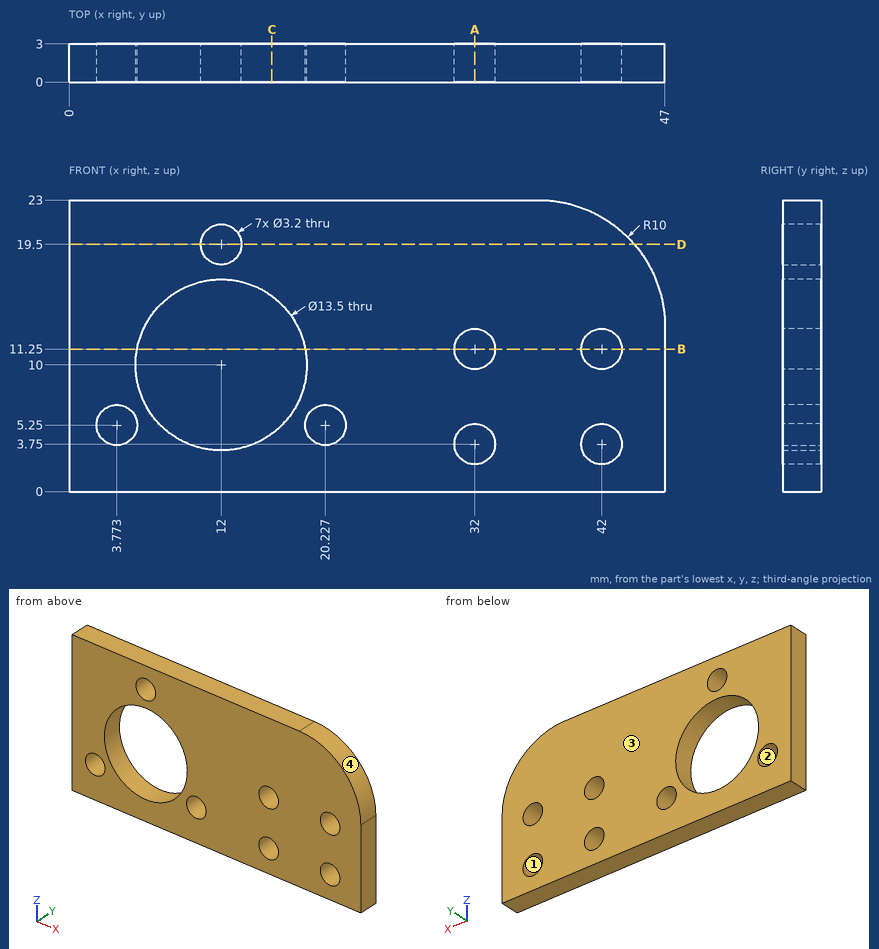
Answer from the drawing. Dimensions are ordinates in mm from the lowest x, y and z of the part. Give positions to 0.01 mm unless a question says otherwise; leave off trailing zeros. Write each loop counter-clockwise with the first axis right and the second up, starting at its lowest first coordinate (ties: lowest second). Pieces come first, ordered by that corner, then holes.
1) Section C-C (x = 16) is taken. Write down the section's boundary in (y, z).
2) Section B-B (z = 11.25) is taken. Write down the section's boundary in (x, y).
3) Given P1, Ø3, axis at x = 32, z = 3.75, coming from the +Y side; P2, Ø3.5, axis at x = 20.23, z = 5.25, coming from the +Y side, each flat-ended and moving along its own axis, determine where each tip first touches the part or whether it passes through.
4) Section D-D (z = 19.5) is taken. Write down the section's boundary in (x, y), and give its area (3 significant figures).
5) Find the intervals of material crossed by L1, parallel to X at y = 2, z = 11.25; L2, parallel to X at y = 2.25, z = 10; L3, parallel to X at y = 2.95, z = 5 (1 decimal), in increasing order.
6) For a pull along X with two mould halves and no side action, classify the marked faces 1, 2, 3 and 4 as pulls with the +X half, pulls with the -X half, needs draft (parallel to the pull), parting line crosses it, or undercut.
7) Section A-A (x = 32) is taken. Write down the section's boundary in (y, z).
Response:
1. outline: (0, 0) - (3, 0) - (3, 4.56) - (0, 4.56) - close; (0, 15.44) - (3, 15.44) - (3, 23) - (0, 23) - close
2. outline: (0, 0) - (5.37, 0) - (5.37, 3) - (0, 3) - close; (18.63, 0) - (30.4, 0) - (30.4, 3) - (18.63, 3) - close; (33.6, 0) - (40.4, 0) - (40.4, 3) - (33.6, 3) - close; (43.6, 0) - (47, 0) - (47, 3) - (43.6, 3) - close
3. P1: passes through
3. P2: stops at y = 3
4. outline: (0, 0) - (10.4, 0) - (10.4, 3) - (0, 3) - close; (13.6, 0) - (44.6, 0) - (44.6, 3) - (13.6, 3) - close
4. area: 124 mm2
5. L1: x = 0 to 5.37, 18.63 to 30.4, 33.6 to 40.4, 43.6 to 47
5. L2: x = 0 to 5.25, 18.75 to 31, 33 to 41, 43 to 47
5. L3: x = 0 to 2.2, 5.4 to 7.5, 16.5 to 18.6, 21.8 to 31, 33 to 41, 43 to 47
6. face 1: undercut
6. face 2: undercut
6. face 3: needs draft
6. face 4: pulls with the +X half
7. outline: (0, 0) - (3, 0) - (3, 2.15) - (0, 2.15) - close; (0, 5.35) - (3, 5.35) - (3, 9.65) - (0, 9.65) - close; (0, 12.85) - (3, 12.85) - (3, 23) - (0, 23) - close
